Build history of the part. All positions in model axes, mm. Face numbers are marked on the shaded views. A direction names the side the tool comes from. Round coordinates to 2 decimals unless told otherwise and drop trailing zeros. Write each loop counter-clockwise with the first axis right and the second up, starting at its lowest first coordinate (ties: lowest second). Pieces come first, ordered by that corner, then holes.
1) Saw through at A-A (y = 103.5). Write the cut outline in (x, z).
2) Saw through at B-B (y = 24). Write the cut outline in (x, z), plus the area to 3 significant figures.
3) Which spindle directions (+Z, -Z, +X, -X, +Y, -Y) get a long thin tool onto all of the face, cutting with end or side? Do the marked faces 1, 2 and 3. Say none if no direction does.
4) Flat gauge pins, fed straight in: pin 1 (2 mm diameter, centred on y = 113, z = -73, fed in from +X); pin 2 (6 mm diameter, centred on x = 0, z = 122, fed in from -Y); pin 3 (8 mm diameter, centred on y = 8, z = 87.5, fed in from -X). Where does each tip first touch, or does it go through?
5) Wall check: probe 1 along Y at (x, z) = (-33, 117); probe 2 along X at (y, z) = (72, 2.5); probe 3 along Z at (x, y) = (7, 9). Give the ranges that are in metal, low to high.
6) Pull direction Z, two halves, no side cores. Call the marked faces 4, 5 and 6: +Z half, -Z half, draft (parallel to the pull), parting line (faces both ways), or undercut.
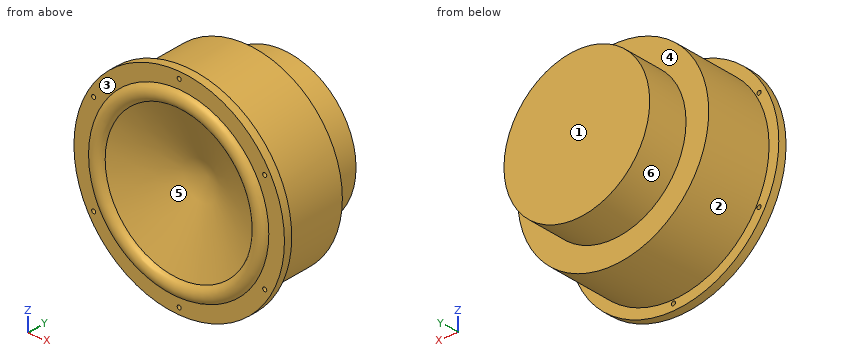
from build123d import *

# Parameters (mm, degrees)
F0_R      = 130
F1_DEPTH  = 10
F2_R      = 118
F3_DEPTH  = 133
F9_D      = 5
F10_R     = 118
F10_R_2   = 90
F11_DEPTH = 50


with BuildPart() as f1:
    # F0 (on Front) → F1 (new body)
    with BuildSketch(Plane.XZ):
        Circle(F0_R)
    extrude(amount=F1_DEPTH)

    # F2 (on face) → F3 (join)
    with BuildSketch(Plane(origin=(0, 0, 0), x_dir=(-1, 0, 0), z_dir=(0, 1, 0))):
        Circle(F2_R)
    extrude(amount=F3_DEPTH)

    # F4 (on Top) → F5 (revolve, cut)
    with BuildSketch(Plane.XY):
        Polygon((0, 0), (0, -40), (160, -40), (0, 30), align=None)
    revolve(axis=Axis((0, -20, 0), (0, 1, 0)), mode=Mode.SUBTRACT)

    # F6 (on Top) → F7 (revolve)
    with BuildSketch(Plane.XY):
        with BuildLine():
            Line((-91.428571, -10), (-110.647532, -10))
            ThreePointArc((-110.647532, -10), (-101.038052, -17.23271), (-91.428571, -10))
        make_face()
    revolve(axis=Axis((0, -10, 0), (0, 1, 0)))

    # F9 (through all)
    with Locations(Plane(origin=(0, 0, 0), x_dir=(-1, 0, 0), z_dir=(0, 1, 0))):
        with Locations((105.655099, 61), (105.655099, -61), (0, -122), (0, 122), (-105.655099, 61), (-105.655099, -61)):
            Hole(F9_D / 2)

    # F10 (on face) → F11 (cut)
    with BuildSketch(Plane(origin=(0, 133, 0), x_dir=(-1, 0, 0), z_dir=(0, 1, 0))):
        Circle(F10_R)
        Circle(F10_R_2, mode=Mode.SUBTRACT)
    extrude(amount=-F11_DEPTH, mode=Mode.SUBTRACT)


solid = f1.part
Evaluation:
1. outline: circle Ø180 at (0, 0)
2. outline: circle Ø236 at (0, 0); hole circle Ø27.43 at (0, 0)
2. area: 43,200 mm2
3. face 1: +Z, -Z, +X, -X, +Y
3. face 2: +Y
3. face 3: -Y
4. pin 1: stops at x = 54
4. pin 2: stops at y = -10
4. pin 3: stops at x = -83.38
5. probe 1: y = -10 to 0
5. probe 2: x = -117.97 to 117.97
5. probe 3: z = -117.79 to -47.49, 47.49 to 117.79
6. face 4: draft
6. face 5: undercut
6. face 6: parting line
